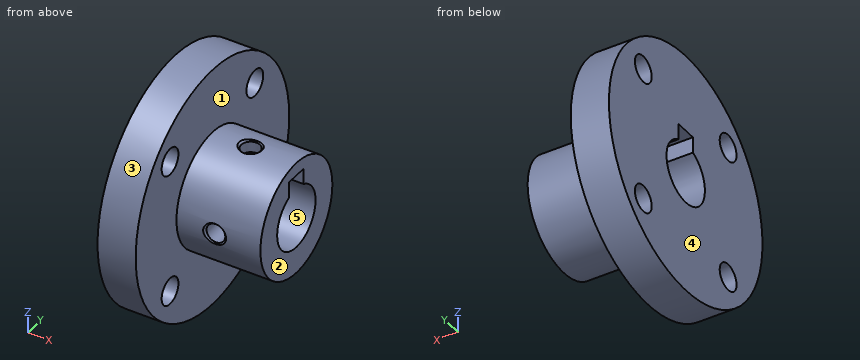
Autodesk Inventor part; units mm, degrees
ref_plane "to_screw1_XY" through (10, 0, 5.8) normal (0, 0, 1) x (1, 0, 0)
ref_plane "to_screw1_YZ" through (10, 0, 5.8) normal (1, 0, 0) x (0, 1, 0)
ref_plane "to_screw1_ZX" through (10, 0, 5.8) normal (0, 1, 0) x (0, 0, 1)
sketch "Sketch_1" plane through (0, 0, 0) normal (0, 0, 1) x (1, 0, 0)
  line L0 (16, 0) -> (0, 0)
  line L1 (0, 4) -> (16, 4)
  line L2 (16, 4) -> (16, 7.5)
  line L3 (16, 7.5) -> (5, 7.5)
  line L4 (5, 7.5) -> (5, 16)
  line L5 (5, 16) -> (0, 16)
  line L6 (0, 16) -> (0, 4)
revolve "Revolution1" add sketch "Sketch_1" angle 360 about axis through (16, 0, 0) along (1, 0, 0)
sketch "Sketch2" plane through (0, 0, 0) normal (-1, 0, 0) x (0, 0, 1)
  point P0 (-8.8388, 8.8388)
hole "Hole1" at (0, 8.8388, -8.8388) direction (1, 0, 0) diameter 3.5 depth 5
pattern_linear "Rectangular Pattern1" count 2 spacing 17.6777 along (0, 0, 1) count 2 spacing 17.6777 along (0, -1, 0) of "Hole1"
sketch "Sketch_4" plane through (10, 0, 0) normal (1, 0, 0) x (0, 0, -1)
  line L0 (0, -7.5) -> (0, -3)
  line L1 (0, -3) -> (1.2295, -3)
  line L2 (1.2295, -3) -> (1.2295, -7.2295)
  line L3 (1.2295, -7.2295) -> (1.5, -7.5)
  line L4 (1.5, -7.5) -> (0, -7.5)
  line L5 (0, -7.5) -> (0, -3)
revolve "Revolution2" cut sketch "Sketch_4" angle 360 about axis through (10, -7.5, 0) along (0, -1, 0)
thread "Thread1"
sketch "Sketch_8" plane through (0, 0, 0) normal (1, 0, 0) x (0, 1, 0)
  line L0 (1.5, 5.8) -> (-1.5, 5.8)
  line L1 (-1.5, 5.8) -> (-1.5, 0)
  line L2 (-1.5, 0) -> (1.5, 0)
  line L3 (1.5, 0) -> (1.5, 5.8)
extrude "Extrusion1" cut sketch "Sketch_8" along normal blind 16
sketch "Sketch_5" plane through (10, 0, 0) normal (1, 0, 0) x (0, 0, -1)
  line L0 (-4, 0) -> (-7.5, 0)
  line L1 (-7.5, 0) -> (-7.5, 1.5)
  line L2 (-7.5, 1.5) -> (-7.2295, 1.2295)
  line L3 (-7.2295, 1.2295) -> (-4, 1.2295)
  line L4 (-4, 1.2295) -> (-4, 0)
  line L5 (-4, 0) -> (-7.5, 0)
revolve "Revolution3" cut sketch "Sketch_5" angle 360 about axis through (10, 0, 4) along (0, 0, -1)
thread "Thread2"
ref_plane "to_screw1_XY" through (10, 0, 5.8) normal (0, 0, 1) x (1, 0, 0)
ref_plane "to_screw1_YZ" through (10, 0, 5.8) normal (1, 0, 0) x (0, 1, 0)
ref_plane "to_screw1_ZX" through (10, 0, 5.8) normal (0, 1, 0) x (0, 0, 1)
ref_plane "to_screw2_XY" through (10, -4, 0) normal (0, -1, 0) x (1, 0, 0)
ref_plane "to_screw2_YZ" through (10, -4, 0) normal (1, 0, 0) x (0, 0, 1)
ref_plane "to_screw2_ZX" through (10, -4, 0) normal (0, 0, 1) x (0, -1, 0)
properties part number "STHRANG8-MB_ss"
Build history of the part. All positions in model axes, mm. Face numbers are marked on the shaded views. A direction names the side the tool comes from. Round coordinates to 2 decimals unless told otherwise and drop trailing zeros. Write each loop counter-clockwise with the first axis right and the second up, starting at its lowest first coordinate (ties: lowest second). Pieces come first, ordered by that corner, then holes. Notation, with made-up numbers: M 72,76.5 L 110,76.5 A32 cw 110,106.5 Z; hole C 2,46 d6. An arc over 180 degrees is marked long. Answer as a JSON object with one key per item and string values. Group by question number.
(1) Flat gauge pins, fed straight in: pin 1 (2 mm diameter, centred on y = -8.84, z = -8.84, fed in from +X); pin 2 (6 mm diameter, centred on y = 11.5, z = 1.5, fed in from +X); pin 3 (3 mm diameter, centred on x = 5.5, z = 12, fed in from -Y); pin 4 (2 mm diameter, centred on x = 8, z = -7, fed in from -Y). Where does each tip first touch, or does it go through?
(2) Cut at B-B (z = 0). Give the cut face in (x, y).
(3) Which spindle directions (+Z, -Z, +X, -X, +Y, -Y) get a long thin tool onto all of the face, cutting with end or side? Do the marked faces 1 and 2. Say none if no direction does.
(4) Mould opens along Y. For the marked faces 3, 4 and 5 say: pulls with the +Y half, pulls with the -Y half, needs draft (parallel to the pull), parting line crosses it, or undercut.
(5) Cut at A-A (y = 0). Give the cut face in (x, z).
(6) Cut at C-C (x = 10). Give the cut face in (y, z), and give its area (3 significant figures).
(7) Cut at D-D (x = 12). Give the cut face in (y, z).
(8) Drill centre lines: L1, parallel to Z at x = 1.5, y = -9; L2, parallel to X at y = -14, z = -1; L3, parallel to X at y = -5.3, z = 0. Where is each one in solid material? Low to high.
Responses:
{
 "1": {"pin 1": "passes through", "pin 2": "stops at x = 5", "pin 3": "stops at y = -12", "pin 4": "stops at y = -4.5"},
 "2": {"outline": "M 0,-16 L 5,-16 L 5,-7.5 L 8.5,-7.5 L 8.77,-7.23 L 8.77,-4 L 0,-4 Z; M 0,4 L 16,4 L 16,7.5 L 5,7.5 L 5,16 L 0,16 Z; M 11.23,-7.23 L 11.5,-7.5 L 16,-7.5 L 16,-4 L 11.23,-4 Z"},
 "3": {"face 1": "+X", "face 2": "+Z, -Z, +X, +Y, -Y"},
 "4": {"face 3": "parting line crosses it", "face 4": "needs draft", "face 5": "undercut"},
 "5": {"outline": "M 0,-16 L 5,-16 L 5,-7.5 L 16,-7.5 L 16,-4 L 0,-4 Z; M 0,5.8 L 8.77,5.8 L 8.77,7.23 L 8.5,7.5 L 5,7.5 L 5,16 L 0,16 Z; M 11.23,5.8 L 16,5.8 L 16,7.5 L 11.5,7.5 L 11.23,7.23 Z"},
 "6": {"outline": "M -7.37,-1.37 A7.5 ccw long 1.37,7.37 L 1.23,7.23 L 1.23,5.8 L 1.5,5.8 L 1.5,3.71 A4 cw long -3.81,-1.23 L -7.23,-1.23 Z; M -7.37,1.37 L -7.23,1.23 L -3.81,1.23 A4 cw -1.5,3.71 L -1.5,5.8 L -1.23,5.8 L -1.23,7.23 L -1.37,7.37 A7.5 ccw Z", "area": "108 mm2"},
 "7": {"outline": "C 0,0 d15; hole M -1.5,3.71 A4 ccw long 1.5,3.71 L 1.5,5.8 L -1.5,5.8 Z"},
 "8": {"L1": "z = -13.23 to -10.58, -7.1 to 7.1, 10.58 to 13.23", "L2": "x = 0 to 5", "L3": "x = 0 to 8.77, 11.23 to 16"}
}
